Work out the finished part from the listing and answer in its coordinate system (mm). A direction names the side the tool comes from. Round coordinates to 2 decimals unless told otherwise and drop trailing zeros. Loops run counter-clockwise (first coordinate to the right, second up) from the corner with the lowest first, then second, coordinate; pieces in that order, holes last. Notation, with made-up numbers: M 8,36.5 L 29,36.5 A28 cw 29,64.5 Z; hole C 60,-11 d2. An arc over 180 degrees is marked long. One line per item, written item: value.
Autodesk Inventor part; units mm, degrees
ref_plane "YZ Plane" through (0, 0, 0) normal (1, 0, 0) x (0, 1, 0)
ref_plane "XZ Plane" through (0, 0, 0) normal (0, 1, 0) x (-1, 0, 0)
ref_plane "XY Plane" through (0, 0, 0) normal (0, 0, 1) x (1, 0, 0)
sketch "スケッチ1" plane through (0, 0, 0) normal (0, 0, 1) x (1, 0, 0)
  circle A0 centre (0, 0) radius 8
  line L0 (-11.2, 0) -> (11.2, 0) construction
  line L1 (0, -11.2) -> (0, 11.2) construction
  circle A1 centre (0, 6) radius 2
  circle A2 centre (0, -6) radius 2
  circle A3 centre (0, 0) radius 1.1
  dimension "d0" = 16
  dimension "d1" = 4
  dimension "d2" = 6
  dimension "d10" = 2.2
extrude "押し出し1" add sketch "スケッチ1" along normal blind 1.5 contours A1 | A2 | A0 | A3
extrude "押し出し2" add sketch "スケッチ1" against normal blind 2.8 contours A1 | A2
chamfer "面取り1" distance 0.3 angle 45 2 edges at (-2, 6, -2.8) (-2, -6, -2.8)
extrude "押し出し3" cut sketch "スケッチ1" along normal blind 10 contours A3
properties part number "adapter_xl320"
1) Find the intervals of material crossed by probe 1 along X at (y, z) = (0, 1.2); probe 2 along Z at (x, y) = (0, 1.25), in increasing order. Write a range as from..to.
Check values:
probe 1: -8..-1.1, 1.1..8
probe 2: 0..1.5
2) The mould has two halves that part along Y. Classify faces 3 (the face through (0, 8, -1)), 4 (the face through (0, -6, -2.8)), 5 (the face through (-1.73, 7.81, 0.74)): +Y half, -Y half, draft (parallel to the pull), parting line (faces both ways), or undercut.
Check values:
face 3: undercut
face 4: draft
face 5: parting line
3) Find section C-C (z = 0.7). Give the vertices of the cut face in (x, y), then the cut area to 3 significant figures.
Check values:
outline: C 0,0 d16; hole C 0,0 d2.2
area: 197 mm2
4) For faces 1 (the face through (0, -8, -1)), 2 (the face through (0, -2, 1.5)), determine the directions among +Z, -Z, +X, -X, +Y, -Y from which every point of the face is accessible in a straight line to the end or side of a thin tool.
Check values:
face 1: -Z
face 2: +Z, +X, -X, +Y, -Y
5) Each of these flat-tipped pins is pushed along its axis until it touches: pin 1 (2 mm diameter, centred on y = 1, z = -1.5, fed in from -X); pin 2 (3 mm diameter, centred on x = 5.5, y = 5, fed in from -Z); pin 3 (3.5 mm diameter, centred on x = 0, y = 0, fed in from +Z); pin 4 (1.5 mm diameter, centred on x = -4, z = -0.5, fed in from -Y). Where does it stop, or does it pass through?
Check values:
pin 1: through
pin 2: z = 0
pin 3: z = 1.5
pin 4: y = -7.22
6) Find section B-B (z = -1.2). Give the vertices of the cut face in (x, y).
Check values:
outline: C 0,-6 d4; C 0,6 d4
7) Find section A-A (y = 0). Give the vertices of the cut face in (x, z).
Check values:
outline: M -8,0 L -1.1,0 L -1.1,1.5 L -8,1.5 Z; M 1.1,0 L 8,0 L 8,1.5 L 1.1,1.5 Z
8) Find section D-D (y = 6). Give the vertices of the cut face in (x, z).
Check values:
outline: M -5.29,0 L -2,0 L -2,-2.5 L -1.7,-2.8 L 1.7,-2.8 L 2,-2.5 L 2,0 L 5.29,0 L 5.29,1.5 L -5.29,1.5 Z
